The listing builds one solid part. Answer for the finished solid, in the listing's coordinates (mm). Coordinates: 2 decimals unless noted, no trailing zeros. Return JSON: item names as keys, results as strings. Group by question number.
1. Find the intervals of material crossed by line 1 along Z through (x, y) = (80, 11); line 2 along Z through (x, y) = (60, 12.75), in increasing order.
2. The mould has two halves that part along Z. Classify faces 1 (the face through (-58.925, 9.86, -78.314)), 2 (the face through (90, 10, 1)), 3 (the face through (-1, 10, 90)): pulls with the +Z half, pulls with the -Z half, needs draft (parallel to the pull), parting line crosses it, or undercut.
3. This flat-tipped pin is pushed along its axis until it touches: P1, Ø3.5, axis at x = 80, z = 60, coming from the -Y side. Where does it stop, or does it pass through?
Autodesk Inventor part; units mm, degrees
ref_plane "YZ Plane" through (0, 0, 0) normal (1, 0, 0) x (0, 1, 0)
ref_plane "XZ Plane" through (0, 0, 0) normal (0, 1, 0) x (-1, 0, 0)
ref_plane "XY Plane" through (0, 0, 0) normal (0, 0, 1) x (1, 0, 0)
sketch "草图2" plane through (0, 0, 0) normal (0, 1, 0) x (-1, 0, 0)
  line L0 (90, 90) -> (-90, 90)
  line L1 (-90, 90) -> (-90, -90)
  line L2 (-90, -90) -> (90, -90)
  line L3 (90, -90) -> (90, 90)
  point P0 (0, 0)
  dimension "d4" = 180
  dimension "d5" = 180
extrude "拉伸2" add sketch "草图2" along normal blind 20
sketch "草图3" plane through (0, 20, 0) normal (0, 1, 0) x (1, 0, 0)
  circle A0 centre (80, 60) radius 2
  point P0 (0, 0)
  dimension "d8" = 4
extrude "拉伸3" cut sketch "草图3" against normal through all
sketch "草图4" plane through (0, 0, 0) normal (0, -1, 0) x (1, 0, 0)
  circle A0 centre (60, -80) radius 2
  point P0 (0, 0)
  dimension "d11" = 4
extrude "拉伸4" cut sketch "草图4" against normal through all
sketch "草图5" plane through (0, 0, 0) normal (0, -1, 0) x (1, 0, 0)
  circle A0 centre (80, 60) radius 2
  point P0 (0, 0)
  dimension "d14" = 4
extrude "拉伸5" cut sketch "草图5" against normal through all
sketch "草图6" plane through (0, 0, 0) normal (0, -1, 0) x (1, 0, 0)
  circle A0 centre (60, 80) radius 2
  point P0 (0, 0)
  dimension "d17" = 4
extrude "拉伸6" cut sketch "草图6" against normal through all
sketch "草图7" plane through (0, 0, 0) normal (0, -1, 0) x (1, 0, 0)
  circle A0 centre (-80, -60) radius 2
  point P0 (0, 0)
  dimension "d20" = 4
extrude "拉伸7" cut sketch "草图7" against normal through all
sketch "草图8" plane through (0, 0, 0) normal (0, -1, 0) x (1, 0, 0)
  circle A0 centre (-60, -80) radius 2
  point P0 (0, 0)
  dimension "d23" = 4
extrude "拉伸8" cut sketch "草图8" against normal through all
sketch "草图9" plane through (0, 0, 0) normal (0, -1, 0) x (1, 0, 0)
  circle A0 centre (-80, 60) radius 2
  point P0 (0, 0)
  dimension "d26" = 4
extrude "拉伸9" cut sketch "草图9" against normal through all
sketch "草图10" plane through (0, 0, 0) normal (0, -1, 0) x (1, 0, 0)
  circle A0 centre (-60, 80) radius 2
  point P0 (0, 0)
  dimension "d29" = 4
extrude "拉伸10" cut sketch "草图10" against normal through all
properties part number "内层升降板"
The answers:
{
 "1": {"line 1": "z = -90 to -62, -58 to 58, 62 to 90", "line 2": "z = -90 to -82, -78 to 78, 82 to 90"},
 "2": {"face 1": "undercut", "face 2": "needs draft", "face 3": "pulls with the +Z half"},
 "3": {"P1": "passes through"}
}
